Could you check a few things on this model? Use its own coordinates, in mm. A direction names the side the tool comes from. Give positions to 0.01 mm unless a question says otherwise; leave off trailing zeros. Order: outer loops, then holes, each group sorted by start corner. A loop starts at its lowest first (then second) coordinate and runs counter-clockwise, first axis right, second up.
(1) Imagine slicing it at C-C, the plane x = 43.5. Write out the boundary of the cut face in (y, z).
(2) Imagine slicing it at B-B, the plane y = -23.5. Write out the boundary of the cut face in (x, z).
(3) If we mould it in two halves opening along X, with no side actions, what happens to faces 5 (the cylindrical face through (42.11, -23.254, 3.219)), 6 (the cylindrical face through (1.91, -29.94, 3.22)), 7 (the cylindrical face through (48.99, -29.84, 3.22)), 8 (the flat face through (25, -16, 0))? For each: released by +X, released by -X, zero draft, split by the parting line, or undercut.
(4) Will these pins go through, and if not, where does the flat tip stop? pin 1 (6 mm diameter, centred on x = 39.5, y = -5.5, fed in from +Z); pin 2 (2 mm diameter, centred on y = -12.5, z = 47.5, fed in from -X); pin 3 (22 mm diameter, centred on x = 32, z = 26.5, fed in from -Y); pin 4 (8 mm diameter, centred on x = 27.5, z = 53, fed in from +Y).
(5) If I drill on probe 1 along Z at (x, y) = (25, -20); probe 2 along Z at (x, y) = (25.4, -10); probe 3 along Z at (x, y) = (27.5, -22), over which ranges is the centre line in solid material (lowest first)?
(6) On a 3-axis mill with a long thin cutter (end or side, diameter ignored), from which of +Z, -Z, +X, -X, +Y, -Y can I reach the whole of each face in a straight line? I mean faces 1 (the flat face through (31.2, -25.4, 47.8)), 2 (the flat face through (38.1, -6, 35)), 3 (the flat face through (12.7, -6, 35)), 4 (the flat face through (26, -22, 6.35)). Say none if no direction works.
(7) Imagine slicing it at A-A, the plane y = -9. Write out the boundary of the cut face in (x, z), then the cut area to 3 significant figures.
(8) Imagine slicing it at D-D, the plane x = 35.5. Write out the boundary of the cut face in (y, z), then the cut area to 3 significant figures.
from build123d import *

# Parameters (mm, degrees)
F0_W      = 50.8
F0_H      = 63.5
F1_DEPTH  = 31.75
F3_DEPTH  = 50.8
F5_DEPTH  = 12.7
F7_DEPTH  = 12.7
F6_R      = 6.35
F8_DEPTH  = 25.4
F9_R      = 3.175
F10_DEPTH = 6.35


with BuildPart() as f1:
    # F0 (on Front) → F1 (new body)
    with BuildSketch(Plane.XZ):
        with Locations((25.4, 31.75)):
            Rectangle(F0_W, F0_H)
    extrude(amount=F1_DEPTH)

    # F2 (on face) → F3 (cut)
    with BuildSketch(Plane.YZ.offset(50.8)):
        Polygon((-31.75, 63.5), (-31.75, 6.35), (-12.7, 6.35), (-12.7, 38.1), (-25.4, 38.1), (-25.4, 63.5), align=None)
    extrude(amount=-F3_DEPTH, mode=Mode.SUBTRACT)

    # F4 (on face) → F5 (cut)
    with BuildSketch(Plane.XZ.offset(12.7)):
        with BuildLine():
            Line((12.7, 19.05), (12.7, 38.1))
            Line((12.7, 38.1), (0, 38.1))
            Line((0, 38.1), (0, 6.35))
            ThreePointArc((0, 6.35), (8.9802561211, 10.0697438789), (12.7, 19.05))
        make_face()
        with BuildLine():
            Line((50.8, 6.35), (50.8, 38.1))
            Line((50.8, 38.1), (38.1, 38.1))
            Line((38.1, 38.1), (38.1, 19.05))
            ThreePointArc((38.1, 19.05), (41.8197438789, 10.0697438789), (50.8, 6.35))
        make_face()
    extrude(amount=-F5_DEPTH, mode=Mode.SUBTRACT)

    # F6 (on face) → F7 (cut)
    with BuildSketch(Plane.XZ.offset(25.4)):
        with BuildLine():
            ThreePointArc((38.1, 50.8), (34.3802561211, 41.8197438789), (25.4, 38.1))
            Line((25.4, 38.1), (38.1, 38.1))
            Line((38.1, 38.1), (38.1, 50.8))
        make_face()
        with BuildLine():
            Line((12.7, 50.8), (12.7, 38.1))
            Line((12.7, 38.1), (25.4, 38.1))
            ThreePointArc((25.4, 38.1), (16.4197438789, 41.8197438789), (12.7, 50.8))
        make_face()
    extrude(amount=-F7_DEPTH, mode=Mode.SUBTRACT)

    # F6 (on face) → F8 (cut)
    with BuildSketch(Plane.XZ.offset(25.4)):
        with Locations((25.4, 50.8)):
            Circle(F6_R)
        Polygon((0, 63.5), (0, 38.1), (12.7, 38.1), (12.7, 50.8), (12.7, 63.5), align=None)
        Polygon((38.1, 63.5), (38.1, 50.8), (38.1, 38.1), (50.8, 38.1), (50.8, 63.5), align=None)
        with BuildLine():
            Line((38.1, 63.5), (25.4, 63.5))
            ThreePointArc((25.4, 63.5), (34.3802561211, 59.7802561211), (38.1, 50.8))
            Line((38.1, 50.8), (38.1, 63.5))
        make_face()
        with BuildLine():
            Line((12.7, 63.5), (12.7, 50.8))
            ThreePointArc((12.7, 50.8), (16.4197438789, 59.7802561211), (25.4, 63.5))
            Line((25.4, 63.5), (12.7, 63.5))
        make_face()
    extrude(amount=-F8_DEPTH, mode=Mode.SUBTRACT)

    # F9 (on face) → F10 (cut)
    with BuildSketch(Plane.XY.offset(6.35)):
        with Locations((6.35, -25.4)):
            Circle(F9_R)
        with Locations((44.45, -25.4)):
            Circle(F9_R)
        with BuildLine():
            ThreePointArc((6.35, -31.75), (1.8598719395, -29.8901280605), (0, -25.4))
            Line((0, -25.4), (0, -31.75))
            Line((0, -31.75), (6.35, -31.75))
        make_face()
        with BuildLine():
            ThreePointArc((50.8, -25.4), (48.9401280605, -29.8901280605), (44.45, -31.75))
            Line((44.45, -31.75), (50.8, -31.75))
            Line((50.8, -31.75), (50.8, -25.4))
        make_face()
    extrude(amount=-F10_DEPTH, mode=Mode.SUBTRACT)


solid = f1.part
Answer block:
1. outline: (-31.75, 0) - (-28.43, 0) - (-28.43, 6.35) - (-31.75, 6.35) - close; (-22.37, 0) - (0, 0) - (0, 8.66) - (-12.7, 8.66) - (-12.7, 6.35) - (-22.37, 6.35) - close
2. outline: (0, 0) - (3.81, 0) - (3.81, 6.35) - (0, 6.35) - close; (8.89, 0) - (41.91, 0) - (41.91, 6.35) - (8.89, 6.35) - close; circle Ø25.4 at (25.4, 50.8); (46.99, 0) - (50.8, 0) - (50.8, 6.35) - (46.99, 6.35) - close; hole circle Ø12.7 at (25.4, 50.8)
3. face 5: undercut
3. face 6: released by -X
3. face 7: released by +X
3. face 8: zero draft
4. pin 1: stops at z = 56.97
4. pin 2: stops at x = 12.7
4. pin 3: stops at y = -12.7
4. pin 4: stops at y = 0
5. probe 1: z = 0 to 6.35, 38.11 to 44.46, 57.14 to 63.49
5. probe 2: z = 0 to 44.45, 57.15 to 63.5
5. probe 3: z = 0 to 6.35, 38.27 to 44.81, 56.79 to 63.33
6. face 1: +Z, +X, -X, -Y
6. face 2: +Z, +X, +Y, -Y
6. face 3: +Z, -X, +Y, -Y
6. face 4: +X, -X, -Y
7. outline: (0, 0) - (50.8, 0) - (50.8, 6.35) arc R12.7 cw to (38.1, 19.05) - (38.1, 50.8) arc R12.7 ccw to (12.7, 50.8) - (12.7, 19.05) arc R12.7 cw to (0, 6.35) - close; hole circle Ø12.7 at (25.4, 50.8)
7. area: 1,650 mm2
8. outline: (-31.75, 0) - (0, 0) - (0, 58.5) - (-25.4, 58.5) - (-25.4, 43.1) - (-12.7, 43.1) - (-12.7, 6.35) - (-31.75, 6.35) - close
8. area: 1,060 mm2
